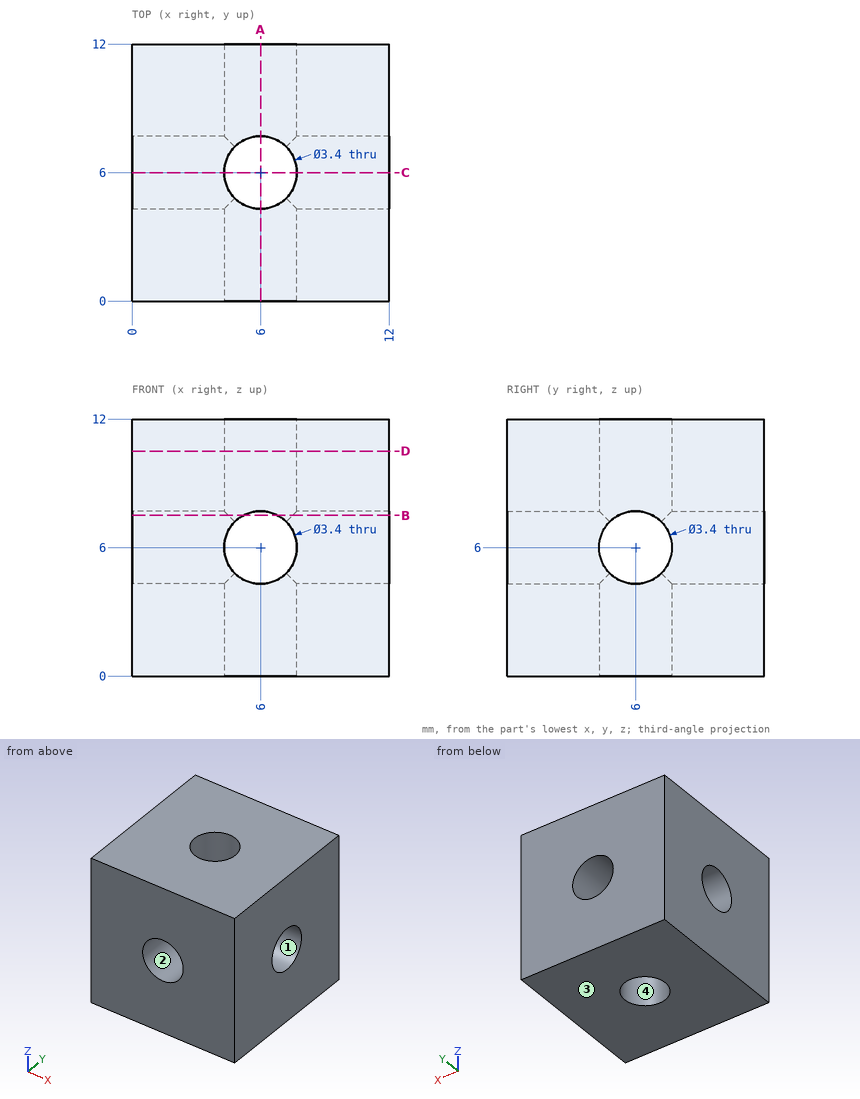
Study the drawing (mm; zero at the part's minimum x, y, z) and answer. Round coordinates to 2 decimals unless told otherwise and drop trailing zeros. Write each loop counter-clockwise with the first axis right and the second up, starting at its lowest first coordinate (ties: lowest second). Pieces come first, ordered by that corner, then holes.
1) The mould has two halves that part along Z. Classify the marked faces 1, 2, 3 and 4: pulls with the +Z half, pulls with the -Z half, needs draft (parallel to the pull), parting line crosses it, or undercut.
2) Given pin 1 Ø3 at (y, z) = (3, 3) entering from -X, flat-ended and moving along its own axis, determine where the tip first touches the part or whether it passes through.
3) A cutting plane is placed at D-D (z = 10.5). Give the vertices of the cut face in (x, y).
4) A straight line is drawn through the part: line 1 (X direction, y = 9.5, z = 6). Find the intervals that lie inside material, in ascending order.
5) A cutting plane is placed at A-A (x = 6). Give the vertices of the cut face in (y, z).
6) A cutting plane is placed at B-B (z = 7.5). Give the vertices of the cut face in (x, y), plus the area to 3 significant figures.
Completed:
1. face 1: undercut
1. face 2: undercut
1. face 3: pulls with the -Z half
1. face 4: needs draft
2. pin 1: stops at x = 0
3. outline: (0, 0) - (12, 0) - (12, 12) - (0, 12) - close; hole circle Ø3.4 at (6, 6)
4. line 1: x = 0 to 4.3, 7.7 to 12
5. outline: (0, 0) - (4.3, 0) - (4.3, 4.3) - (0, 4.3) - close; (0, 7.7) - (4.3, 7.7) - (4.3, 12) - (0, 12) - close; (7.7, 0) - (12, 0) - (12, 4.3) - (7.7, 4.3) - close; (7.7, 7.7) - (12, 7.7) - (12, 12) - (7.7, 12) - close
6. outline: (0, 0) - (5.2, 0) - (5.2, 4.5) arc R1.7 cw to (4.5, 5.2) - (0, 5.2) - close; (0, 6.8) - (4.5, 6.8) arc R1.7 cw to (5.2, 7.5) - (5.2, 12) - (0, 12) - close; (6.8, 0) - (12, 0) - (12, 5.2) - (7.5, 5.2) arc R1.7 cw to (6.8, 4.5) - close; (6.8, 7.5) arc R1.7 cw to (7.5, 6.8) - (12, 6.8) - (12, 12) - (6.8, 12) - close
6. area: 107 mm2
